```python
from build123d import *

# Parameters (mm, degrees)
F0_W      = 13
F0_H      = 13
F1_DEPTH  = 16
F3_D      = 10.8
F4_R      = 7.5
F5_DEPTH  = 30.5
F6_R      = 6.9
F7_DEPTH  = 1
F8_R      = 6.75
F9_DEPTH  = 9.8
F10_R     = 2.5
F11_DEPTH = 50
F12_R     = 10
F12_W     = 13
F12_H     = 13
F13_DEPTH = 16
F15_DEPTH = 25


with BuildPart() as f1:
    # F0 (on Top) → F1 (new body)
    with BuildSketch(Plane.XY):
        Rectangle(F0_W, F0_H)
    extrude(amount=F1_DEPTH)

    # F3 (through all)
    with Locations(Plane(origin=(0, 0, 0), x_dir=(1, 0, 0), z_dir=(0, 0, -1))):
        with Locations((0, 0)):
            Hole(F3_D / 2)

    # F4 (on face) → F5 (join)
    with BuildSketch(Plane.XY.offset(16)):
        Circle(F4_R)
    extrude(amount=F5_DEPTH)

    # F6 (on face) → F7 (cut)
    with BuildSketch(Plane.XY.offset(46.5)):
        Circle(F6_R)
    extrude(amount=-F7_DEPTH, mode=Mode.SUBTRACT)

    # F8 (on face) → F9 (cut)
    with BuildSketch(Plane.XY.offset(45.5)):
        Circle(F8_R)
    extrude(amount=-F9_DEPTH, mode=Mode.SUBTRACT)

    # F10 (on face) → F11 (cut)
    with BuildSketch(Plane.XY.offset(35.7)):
        Circle(F10_R)
    extrude(amount=-F11_DEPTH, mode=Mode.SUBTRACT)

    # F12 (on face) → F13 (join, through all)
    with BuildSketch(Plane(origin=(0, 0, 0), x_dir=(1, 0, 0), z_dir=(0, 0, -1))):
        Circle(F12_R)
        Rectangle(F12_W, F12_H, mode=Mode.SUBTRACT)
    extrude(amount=-F13_DEPTH)

    # F14 (on face) → F15 (cut)
    with BuildSketch(Plane(origin=(0, 0, 0), x_dir=(1, 0, 0), z_dir=(0, 0, -1))):
        with BuildLine():
            ThreePointArc((4.8412291828, 8.75), (0, 10), (-4.8412291828, 8.75))
            Line((-4.8412291828, 8.75), (4.8412291828, 8.75))
        make_face()
        with BuildLine():
            Line((4.8412291828, -8.75), (-4.8412291828, -8.75))
            ThreePointArc((-4.8412291828, -8.75), (0, -10), (4.8412291828, -8.75))
        make_face()
    extrude(amount=-F15_DEPTH, mode=Mode.SUBTRACT)


solid = f1.part
```
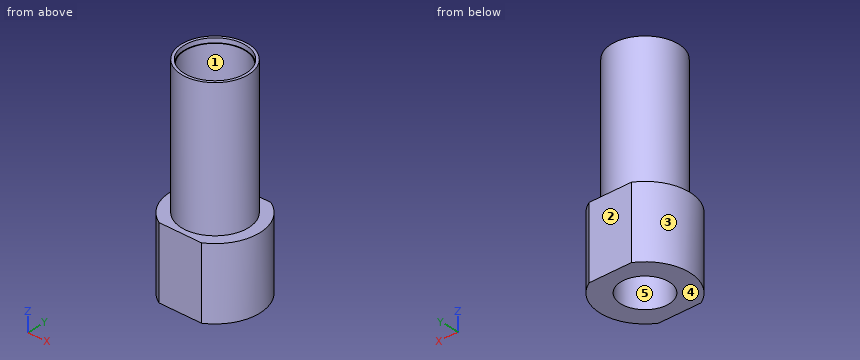
The listing builds one solid part. Answer for the finished solid, in the listing's coordinates (mm). Face numbers are marked on the shaded views. A direction names the side the tool comes from. Coordinates: 2 decimals unless noted, no trailing zeros. Loops run counter-clockwise (first coordinate to the right, second up) from the corner with the lowest first, then second, coordinate; pieces in that order, holes last. Notation, with made-up numbers: M 15.5,56 L 65.5,56 A15 ccw 65.5,60 Z; hole C -39.75,11.5 d11. An arc over 180 degrees is marked long. Answer as a JSON object with one key per item and string values. Group by question number.
Item 1: Each of these flat-tipped pins is pushed along its axis until it touches: P1, Ø9.5, axis at x = 0, y = 0, coming from the -Z side; P2, Ø7, axis at x = -0.5, y = -2, coming from the +Z side; P3, Ø2, axis at x = 6.5, z = 15.5, coming from the +Y side. Where does it stop, or does it pass through?
Item 2: Section D-D (y = -6) is taken. Write down the section's boundary in (x, z).
Item 3: Section C-C (z = 3.5) is taken. Write down the section's boundary in (x, y).
Item 4: Which of the six approach directions +Z, -Z, +X, -X, +Y, -Y give full straight-line access (tool end or side, diameter ignored) to the marked faces 1 and 2?
Item 5: Section B-B (y = 0) is taken. Write down the section's boundary in (x, z), and give its area (3 significant figures).
Item 6: Section A-A (x = 0) is taken. Write down the section's boundary in (y, z), and give its area (3 significant figures).
Item 7: Consider L1, parallel to Y at x = 0, z = 7.75; L2, parallel to Y at x = 0, z = 30.75; L3, parallel to Z at x = -8, y = 5. Determine where each line is inside the solid, lowest interval first.
Item 8: Determine the mould class of the marked faces 3, 4 and 5 for opening direction Y: +Y half, -Y half, draft (parallel to the pull), parting line (faces both ways), or undercut.
Solved:
{
 "1": {"P1": "stops at z = 16", "P2": "stops at z = 35.7", "P3": "stops at y = 8.35"},
 "2": {"outline": "M -8,0 L 8,0 L 8,16 L 4.5,16 L 4.5,46.5 L 3.41,46.5 L 3.41,45.5 L 3.09,45.5 L 3.09,35.7 L -3.09,35.7 L -3.09,45.5 L -3.41,45.5 L -3.41,46.5 L -4.5,46.5 L -4.5,16 L -8,16 Z"},
 "3": {"outline": "M -4.84,-8.75 L 4.84,-8.75 A10 ccw 4.84,8.75 L -4.84,8.75 A10 ccw Z; hole C 0,0 d10.8"},
 "4": {"face 1": "+Z", "face 2": "+Z, -Z, +X, -X, +Y"},
 "5": {"outline": "M -10,0 L -5.4,0 L -5.4,16 L -2.5,16 L -2.5,35.7 L -6.75,35.7 L -6.75,45.5 L -6.9,45.5 L -6.9,46.5 L -7.5,46.5 L -7.5,16 L -10,16 Z; M 2.5,16 L 5.4,16 L 5.4,0 L 10,0 L 10,16 L 7.5,16 L 7.5,46.5 L 6.9,46.5 L 6.9,45.5 L 6.75,45.5 L 6.75,35.7 L 2.5,35.7 Z", "area": "360 mm2"},
 "6": {"outline": "M -8.75,0 L -5.4,0 L -5.4,16 L -2.5,16 L -2.5,35.7 L -6.75,35.7 L -6.75,45.5 L -6.9,45.5 L -6.9,46.5 L -7.5,46.5 L -7.5,16 L -8.75,16 Z; M 2.5,16 L 5.4,16 L 5.4,0 L 8.75,0 L 8.75,16 L 7.5,16 L 7.5,46.5 L 6.9,46.5 L 6.9,45.5 L 6.75,45.5 L 6.75,35.7 L 2.5,35.7 Z", "area": "320 mm2"},
 "7": {"L1": "y = -8.75 to -5.4, 5.4 to 8.75", "L2": "y = -7.5 to -2.5, 2.5 to 7.5", "L3": "z = 0 to 16"},
 "8": {"face 3": "parting line", "face 4": "draft", "face 5": "undercut"}
}
